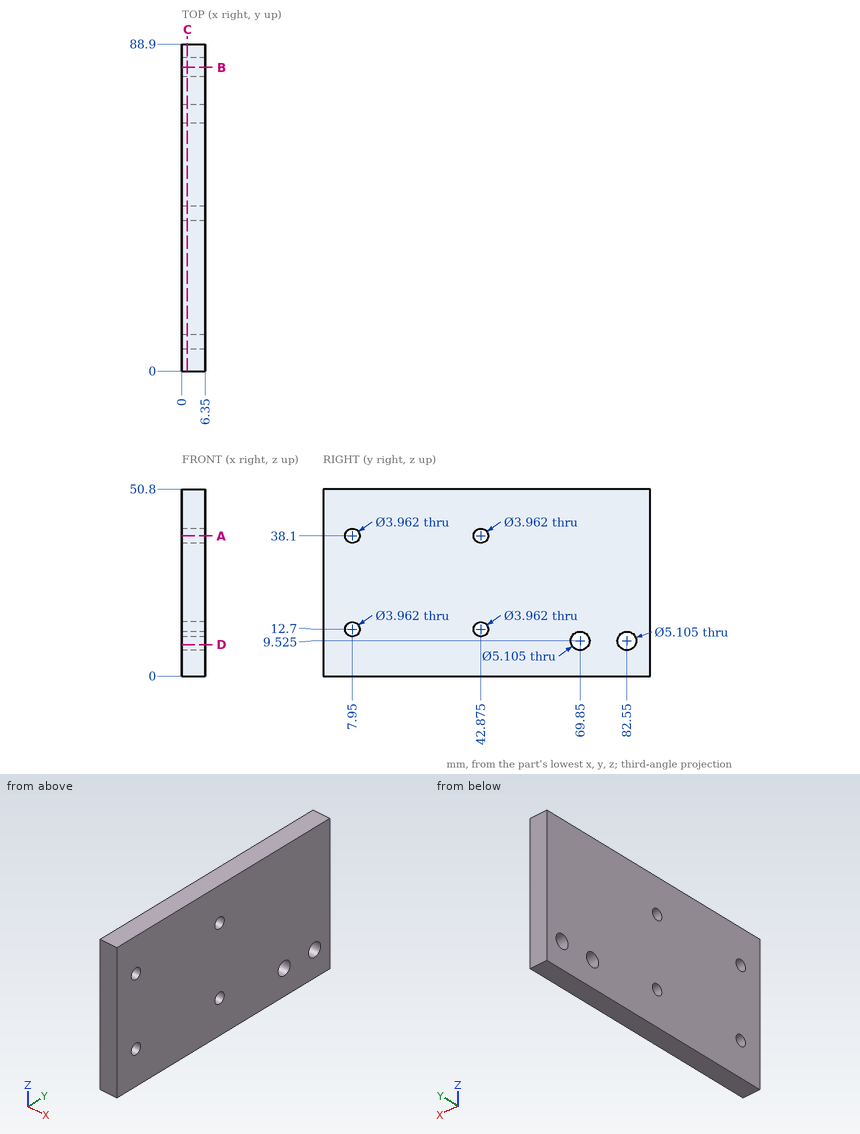
Can you work these out from the drawing? Everything is in mm from the part's minimum corner. Give positions to 0.01 mm unless a question says otherwise; leave off trailing zeros. Order: outer loops, then holes, each group sorted by start corner. A loop starts at its lowest first (then second) coordinate and runs counter-clockwise, first axis right, second up.
Item 1: If we section it at C-C, the plane x = 1.5: Count the separate pieces of the cut face and the enclosed holes in it, plus the area to 3 significant figures.
Item 2: If we section it at B-B, the plane y = 82.55: Write out the boundary of the cut face in (x, z).
Item 3: If we section it at D-D, the plane z = 8.5: Write out the boundary of the cut face in (x, y), plus the area to 3 significant figures.
Item 4: I need wall thicknesses on line 1 (Y direction, x = 3.25, z = 38.1); line 2 (Z direction, x = 3.5, y = 69.85); line 3 (Y direction, x = 1, z = 8.5). Which ranges of each line are inside material? Lowest first, please.
Item 5: If we section it at A-A, the plane z = 38.1: Write out the boundary of the cut face in (x, y), plus the area to 3 significant figures.
Values:
1. separate pieces: 1
1. enclosed holes: 6
1. area: 4,430 mm2
2. outline: (0, 0) - (6.35, 0) - (6.35, 6.97) - (0, 6.97) - close; (0, 12.08) - (6.35, 12.08) - (6.35, 50.8) - (0, 50.8) - close
3. outline: (0, 0) - (6.35, 0) - (6.35, 67.51) - (0, 67.51) - close; (0, 72.19) - (6.35, 72.19) - (6.35, 80.21) - (0, 80.21) - close; (0, 84.89) - (6.35, 84.89) - (6.35, 88.9) - (0, 88.9) - close
3. area: 505 mm2
4. line 1: y = 0 to 5.97, 9.93 to 40.89, 44.86 to 88.9
4. line 2: z = 0 to 6.97, 12.08 to 50.8
4. line 3: y = 0 to 67.51, 72.19 to 80.21, 84.89 to 88.9
5. outline: (0, 0) - (6.35, 0) - (6.35, 5.97) - (0, 5.97) - close; (0, 9.93) - (6.35, 9.93) - (6.35, 40.89) - (0, 40.89) - close; (0, 44.86) - (6.35, 44.86) - (6.35, 88.9) - (0, 88.9) - close
5. area: 514 mm2
